Geometry check sheet. Reference: the model listing, model coordinates, mm. A direction names the side the tool comes from. Round coordinates to 2 decimals unless told otherwise and drop trailing zeros. Order: outer loops, then holes, each group sorted by start corner. A loop starts at its lowest first (then second) coordinate and runs counter-clockwise, first axis right, second up. Notation, with made-up numbers: (37.5, -31) -> (42.5, -31) arc R26 cw to (42.5, 1) -> close; hole circle Ø10 at (36, -25). An arc over 180 degrees is marked (long way). Use a Markdown table: item, result. Add a question column.
Item 1: Sectioned sample at A-A, the plane z = 23.5. Record the cut outline in (x, y), and give its area (3 significant figures).
Item 2: Gauge pin test, flat ends, axial feed: pin 1 Ø10 at (y, z) = (41.5, 39) entering from +X; pin 2 Ø6 at (x, z) = (28, 26) entering from +Y; pin 3 Ø5 at (x, z) = (12.5, 38) entering from +Y. Record the tip position at first contact, or that the pin passes through.
Item 3: Material ranges on probe 1 along Z at (x, y) = (-6, 23); probe 2 along Y at (x, z) = (-9.5, 13); probe 3 along Z at (x, y) = (-2, 33), recorded low to high. Write a range as [from, to].
Item 4: Sectioned sample at C-C, the plane z = 34. Record the cut outline in (x, y), and give its area (3 significant figures).
Item 5: Sectioned sample at D-D, the plane y = 9.5. Record the cut outline in (x, z).
Item 6: Sectioned sample at B-B, the plane y = 52. Record the cut outline in (x, z).
Item 7: Mould release check, pull along X, two halves, no side actions. Record for faces 4 (the flat face through (17.11, 21.73, 31.02)), 5 (the flat face through (-12.025, 19.49, 28.906)), 6 (the flat face through (-3, 23, 56.642)): pulls with the +X half, pulls with the -X half, needs draft (parallel to the pull), parting line crosses it, or undercut.
Item 8: Set-up check for faces 1 (the flat face through (8, 41, 6.096)), 2 (the flat face through (-11, 56.892, 31)), 3 (the flat face through (-22.167, 34, 28)): record each of +Z, -Z, +X, -X, +Y, -Y from which the full face is reachable in a straight line by a thin tool's end or side.
from build123d import *

# Parameters (mm, degrees)
F0_W     = 22.1668612212
F0_H     = 66.4054453373
F1_DEPTH = 6.096
F3_DEPTH = 50.546
F4_R     = 9.1249243662
F5_DEPTH = 27.178


with BuildPart() as f1:
    # F0 (on Top) → F1 (new body)
    with BuildSketch(Plane.XY):
        Polygon((0, 66.4054453373), (0, 0), (34.1540910304, 0), align=None)
        with Locations((-11.0834306106, 33.2027226686)):
            Rectangle(F0_W, F0_H)
    extrude(amount=F1_DEPTH)

    # F2 (on face) → F3 (join)
    with BuildSketch(Plane.XY.offset(6.096)):
        Polygon((0, 56.8917728961), (-22.1668612212, 56.8917728961), (-22.1668612212, 0), (27.6847910136, 0), align=None)
    extrude(amount=F3_DEPTH)

    # F4 (on face) → F5 (cut)
    with BuildSketch(Plane(origin=(22.3841916607, 10.892641178, 0), x_dir=(-0.4375642832, 0.8991871318, 0), z_dir=(0.8991871318, 0.4375642832, 0))):
        with Locations((22.9144543409, 28.7781264633)):
            Circle(F4_R)
    extrude(amount=-F5_DEPTH, mode=Mode.SUBTRACT)


solid = f1.part
Found:
| question | item | result |
|---|---|---|
| 1 | outline | (-22.17, 0) -> (27.68, 0) -> (15.61, 24.8) -> (-8.82, 12.91) -> (-15.34, 26.3) -> (9.1, 38.19) -> (0, 56.89) -> (-22.17, 56.89) -> close |
| 1 | area | 1,640 mm2 |
| 2 | pin 1 | stops at x = 9.92 |
| 2 | pin 2 | stops at y = 5.52 |
| 2 | pin 3 | stops at y = 36.34 |
| 3 | probe 1 | z = [0, 19.66], [37.89, 56.64] |
| 3 | probe 2 | y = [0, 56.89] |
| 3 | probe 3 | z = [0, 23.78], [33.78, 56.64] |
| 4 | outline | (-22.17, 0) -> (27.68, 0) -> (15.63, 24.77) -> (-8.81, 12.88) -> (-15.35, 26.33) -> (9.08, 38.23) -> (0, 56.89) -> (-22.17, 56.89) -> close |
| 4 | area | 1,640 mm2 |
| 5 | outline | (-22.17, 0) -> (29.27, 0) -> (29.27, 6.1) -> (23.06, 6.1) -> (23.06, 56.64) -> (-22.17, 56.64) -> close |
| 6 | outline | (-22.17, 0) -> (7.41, 0) -> (7.41, 6.1) -> (2.38, 6.1) -> (2.38, 56.64) -> (-22.17, 56.64) -> close |
| 7 | face 4 | pulls with the +X half |
| 7 | face 5 | undercut |
| 7 | face 6 | needs draft |
| 8 | face 1 | +Z, +X, +Y |
| 8 | face 2 | +Z, +X, -X, +Y |
| 8 | face 3 | +Z, -Z, -X, +Y, -Y |
